Verification items for this drawing (mm, ordinates from the low corner). A direction names the side the tool comes from. Coordinates: 2 decimals unless noted, no trailing zeros. Order: outer loops, then holes, each group sorted by start corner. A loop starts at its lowest first (then second) coordinate and runs counter-clockwise, first axis right, second up.
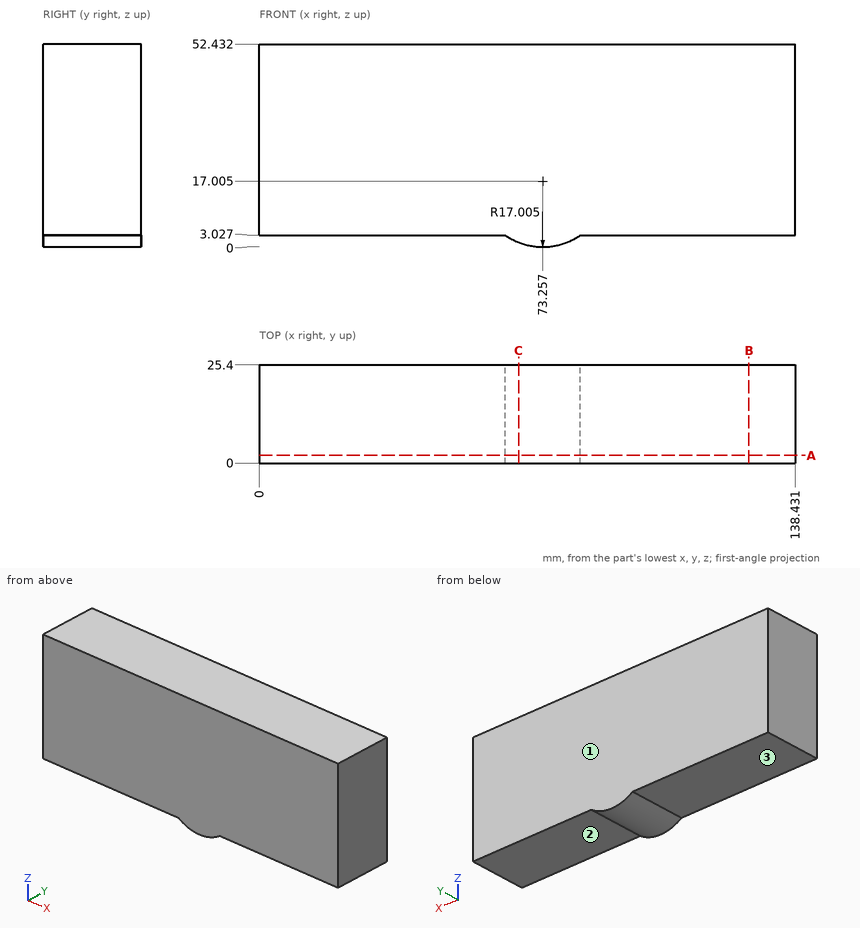
(1) Cross-section at A-A (y = 2). Enter the section's corners in (x, z) (1 decimal).
Filled in:
outline: (0, 3) - (63.6, 3) arc R17 ccw to (82.9, 3) - (138.4, 3) - (138.4, 52.4) - (0, 52.4) - close
(2) Go/stop test with flat-tipped pins: P1, Ø8, axis at x = 22.5, y = 5.5, coming from the -Z side; P2, Ø12, axis at x = 81.5, y = 21.5, coming from the -Z side. Record where each tip stops, or that it passes through.
Filled in:
P1: stops at z = 3.03
P2: stops at z = 0.15
(3) Cross-section at C-C (x = 67). Enter the section's corners in (y, z), and give its area (3 significant figures).
Filled in:
outline: (0, 1.19) - (25.4, 1.19) - (25.4, 52.43) - (0, 52.43) - close
area: 1,300 mm2
(4) Cross-section at B-B (x = 126.5). Enter the section's corners in (y, z), and give its area (4 significant figures).
Filled in:
outline: (0, 3.03) - (25.4, 3.03) - (25.4, 52.43) - (0, 52.43) - close
area: 1,255 mm2
(5) Tool access check on the marked faces 1, 2 and 3. Record the directions out of +Z, -Z, +X, -X, +Y, -Y that give a thin tool (end or side, any length) a straight path to the whole face; none if there is none.
Filled in:
face 1: +Z, -Z, +X, -X, +Y
face 2: -Z, +X, +Y, -Y
face 3: -Z, -X, +Y, -Y
(6) Thickness scan on probe 1 along Z at (x, y) = (23.5, 24.25); probe 2 along Z at (x, y) = (76.5, 16.75). Record the ranges inside material, lowest first.
Filled in:
probe 1: z = 3.03 to 52.43
probe 2: z = 0.31 to 52.43
